For this review, take the finished solid that the model builds, in its own axes (mm). A direction names the side the tool comes from. Round coordinates to 2 decimals unless told otherwise and drop trailing zeros. Loops run counter-clockwise (first coordinate to the right, second up) from the corner with the lowest first, then second, coordinate; pieces in that order, holes last.
1) Tool access review of faces 1 (the cylindrical face through (0.41, 38.82, 30.07)), 2 (the cylindrical face through (16.983, 38.71, 30.073)), 3 (the flat face through (1, -15, -2)), 4 (the cylindrical face through (-15.475, -15.232, 30.073)), 5 (the cylindrical face through (19.64, -5.95, 30.07)): name each direction out of +Z, -Z, +X, -X, +Y, -Y from which nothing blocks a thin tool from reaching the whole face with its end or side.
2) Insertion check: pin 1 (12 mm diameter, centred on y = -59.5, z = 21.5, fed in from +X); pin 2 (5 mm diameter, centred on y = 28, z = 30.5, fed in from -X); pin 3 (1 mm diameter, centred on y = -63, z = 25, fed in from -X). Each pin has a flat end and moves straight along its axis. Give the tip position at first contact, or say it passes through.
3) Wall thickness on L1, parallel to Y at x = 10.5, z = 30; L2, parallel to Y at x = 0, z = 52.5; L3, parallel to X at y = 22, z = 46: over which ranges is each line inside the solid? List them lowest first.
4) Mouldability with a two-part tool opening along Y and no side actions: class faces 6 (the cylindrical face through (16.836, -34.443, 30.073)), 7 (the flat face through (0, -15, 61)), 8 (the cylindrical face through (0.607, -69.613, 30.073)) as pulls with the +Y half, pulls with the -Y half, needs draft (parallel to the pull), parting line crosses it, or undercut.
5) Take a section at B-B (x = 3). State the section outline as (y, z) points.
6) Take a section at A-A (y = -27). State the section outline as (x, z) points.
7) Take a section at C-C (z = 56.5). State the section outline as (x, y) points.
```python
from build123d import *

# Parameters (mm, degrees)
EXTRUDE1_DEPTH = 61
SKETCH2_W      = 40.918085351
SKETCH2_H      = 123.5
EXTRUDE6_DEPTH = 2


with BuildPart() as part:
    # Sketch1 → Extrude1 (new body)
    with BuildSketch(Plane.XY):
        with BuildLine():
            ThreePointArc((18.117441581, 26.964443994), (16.856617983, 38.839101272), (4.981960705, 40.09992487))
            ThreePointArc((4.981960705, 40.09992487), (0.344560099, 38.823949387), (-4.1863741, 40.437713029))
            ThreePointArc((-4.1863741, 40.437713029), (-15.67064328, 38.66031776), (-16.842423207, 27.098548676))
            ThreePointArc((-16.842423207, 27.098548676), (-15.474586856, 22.702284028), (-16.756389299, 18.280168965))
            ThreePointArc((-16.756389299, 18.280168965), (-18.278642652, 13.201858254), (-16.842423207, 8.098548676))
            ThreePointArc((-16.842423207, 8.098548676), (-15.474586856, 3.702284028), (-16.756389299, -0.719831035))
            ThreePointArc((-16.756389299, -0.719831035), (-18.278642652, -5.798141746), (-16.842423207, -10.901451324))
            ThreePointArc((-16.842423207, -10.901451324), (-15.474586856, -15.297715972), (-16.756389299, -19.719831035))
            ThreePointArc((-16.756389299, -19.719831035), (-18.278642652, -24.798141746), (-16.842423207, -29.901451324))
            ThreePointArc((-16.842423207, -29.901451324), (-15.474586856, -34.297715972), (-16.756389299, -38.719831035))
            ThreePointArc((-16.756389299, -38.719831035), (-18.278642652, -43.798141746), (-16.842423207, -48.901451324))
            ThreePointArc((-16.842423207, -48.901451324), (-15.474586856, -53.297715972), (-16.756389299, -57.719831035))
            ThreePointArc((-16.756389299, -57.719831035), (-15.510318105, -69.582077178), (-3.653305695, -70.877003311))
            ThreePointArc((-3.653305695, -70.877003311), (0.671232667, -69.612662366), (4.993176556, -70.885843854))
            ThreePointArc((4.993176556, -70.885843854), (16.87201709, -69.603985894), (18.117441581, -57.721270292))
            ThreePointArc((18.117441581, -57.721270292), (16.836042019, -53.378413149), (18.117441581, -49.035556006))
            ThreePointArc((18.117441581, -49.035556006), (19.639103562, -43.878413149), (18.117441581, -38.721270292))
            ThreePointArc((18.117441581, -38.721270292), (16.836042019, -34.378413149), (18.117441581, -30.035556006))
            ThreePointArc((18.117441581, -30.035556006), (19.639103562, -24.878413149), (18.117441581, -19.721270292))
            ThreePointArc((18.117441581, -19.721270292), (16.836042019, -15.378413149), (18.117441581, -11.035556006))
            ThreePointArc((18.117441581, -11.035556006), (19.639103562, -5.878413149), (18.117441581, -0.721270292))
            ThreePointArc((18.117441581, -0.721270292), (16.836042019, 3.621586851), (18.117441581, 7.964443994))
            ThreePointArc((18.117441581, 7.964443994), (19.639103562, 13.121586851), (18.117441581, 18.278729708))
            ThreePointArc((18.117441581, 18.278729708), (16.836042019, 22.621586851), (18.117441581, 26.964443994))
        make_face()
    extrude(amount=EXTRUDE1_DEPTH)

    # Sketch2 → Extrude6 (add)
    with BuildSketch(Plane(origin=(0, 0, 0), x_dir=(-1, 0, 0), z_dir=(0, 0, -1))):
        with Locations((-0.680060887, -15.628413149)):
            Rectangle(SKETCH2_W, SKETCH2_H)
    extrude(amount=EXTRUDE6_DEPTH)


solid = part.part
```
Response:
1. face 1: +Z, +Y
1. face 2: +Z
1. face 3: -Z, +X, -X, +Y, -Y
1. face 4: +Z, -X
1. face 5: +Z, +X
2. pin 1: stops at x = 19.65
2. pin 2: stops at x = -18.14
2. pin 3: stops at x = -18.28
3. L1: y = -72.39 to 41.61
3. L2: y = -69.64 to 38.84
3. L3: x = -15.5 to 16.86
4. face 6: undercut
4. face 7: needs draft
4. face 8: pulls with the -Y half
5. outline: (-77.38, -2) - (46.12, -2) - (46.12, 0) - (39.17, 0) - (39.17, 61) - (-69.96, 61) - (-69.96, 0) - (-77.38, 0) - close
6. outline: (-19.78, -2) - (21.14, -2) - (21.14, 0) - (19.4, 0) - (19.4, 61) - (-18.04, 61) - (-18.04, 0) - (-19.78, 0) - close
7. outline: (-16.84, -48.9) arc R8 cw to (-16.76, -57.72) arc R9.5 ccw to (-3.65, -70.88) arc R8 cw to (4.99, -70.89) arc R9.51 ccw to (18.12, -57.72) arc R8 cw to (18.12, -49.04) arc R9.5 ccw to (18.12, -38.72) arc R8 cw to (18.12, -30.04) arc R9.5 ccw to (18.12, -19.72) arc R8 cw to (18.12, -11.04) arc R9.5 ccw to (18.12, -0.72) arc R8 cw to (18.12, 7.96) arc R9.5 ccw to (18.12, 18.28) arc R8 cw to (18.12, 26.96) arc R9.5 ccw to (4.98, 40.1) arc R8 cw to (-4.19, 40.44) arc R9.5 ccw to (-16.84, 27.1) arc R8 cw to (-16.76, 18.28) arc R9.5 ccw to (-16.84, 8.1) arc R8 cw to (-16.76, -0.72) arc R9.5 ccw to (-16.84, -10.9) arc R8 cw to (-16.76, -19.72) arc R9.5 ccw to (-16.84, -29.9) arc R8 cw to (-16.76, -38.72) arc R9.5 ccw to start
